Geometry: final body of the model. Coordinates: model frame, mm. Give positions to 0.01 mm unless a question says otherwise; leave off trailing zeros. Write each loop counter-clockwise with the first axis right and the second up, starting at its lowest first coordinate (ties: lowest second). Pieces come first, ordered by that corner, then holes. Notation, with made-up numbers: M 42,75.25 L 52,75.25 A22 cw 52,98.25 Z; hole C -20,86 d3. An arc over 180 degrees is marked long. One line per question, with ' | ' between items.
from build123d import *

# Parameters (mm, degrees)
F0_W     = 914.4
F0_H     = 762
F1_DEPTH = 609.6
F3_W     = 914.4
F3_H     = 762
F4_DEPTH = 609.6
F6_DEPTH = 2057.04989884
F8_DEPTH = 609.601


with BuildPart() as f1:
    # F0 (on Front) → F1 (new body)
    with BuildSketch(Plane.XZ):
        with Locations((-0.35110116, 123.4715153943)):
            Rectangle(F0_W, F0_H)
    extrude(amount=F1_DEPTH)


with BuildPart() as f1_1:
    # F2: moved
    add(f1.part.moved(Location((1143, 0, 0))))

    # F5 (on face) → F6 (cut, through all)
    with BuildSketch(Plane.YZ.offset(1599.84889884)):
        with BuildLine():
            Line((-609.6, 504.4715153943), (-609.6, -143.2284846057))
            ThreePointArc((-609.6, -143.2284846057), (-393.902496237, 149.2118568345), (-317.5, 504.4715153943))
            Line((-317.5, 504.4715153943), (-609.6, 504.4715153943))
        make_face()
    extrude(amount=-F6_DEPTH, mode=Mode.SUBTRACT)


with BuildPart() as f4:
    # F3 (on Front) → F4 (new body)
    with BuildSketch(Plane.XZ):
        Rectangle(F3_W, F3_H)
    extrude(amount=F4_DEPTH)

    # F7 (on face) → F8 (cut, through all)
    with BuildSketch(Plane.XZ.offset(609.6)):
        with BuildLine():
            Line((-457.2, 381), (-457.2, -266.7))
            ThreePointArc((-457.2, -266.7), (-287.4268495342, 37.5712410121), (-228.6, 381))
            Line((-228.6, 381), (-457.2, 381))
        make_face()
        with BuildLine():
            Line((457.2, 381), (228.6, 381))
            ThreePointArc((228.6, 381), (287.4268495342, 37.5712410121), (457.2, -266.7))
            Line((457.2, -266.7), (457.2, 381))
        make_face()
    extrude(amount=-F8_DEPTH, mode=Mode.SUBTRACT)


with BuildPart() as f1_2:
    # F9: moved
    add(f1_1.part.moved(Location((-1143, 0, -123.2408))))

    # F10: intersect F4
    add(f4.part, mode=Mode.INTERSECT)


solid = f1_2.part
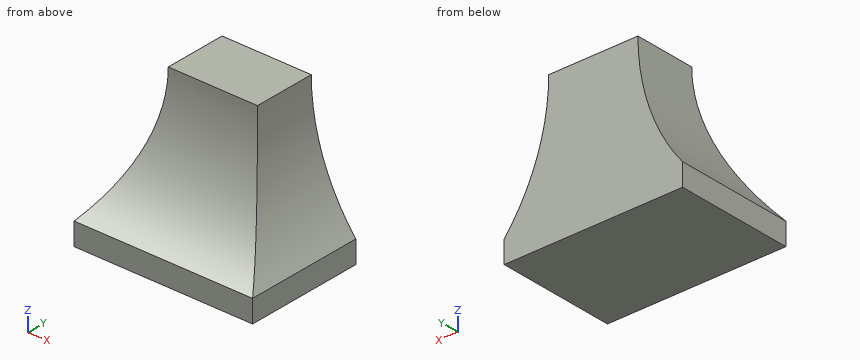
(1) Cut plane B-B, the plane y = -127. Return loops of the section in (x, z) (3 decimals), then the cut area to 3 significant figures.
Working result:
outline: M -457.2,-380.769 L 456.849,-380.769 L 456.849,-266.264 A1031.875 cw 228.6,381 L -228.6,381 A1031.875 cw -457.2,-266.7 Z | area: 494,000 mm^2
(2) Material intervals for L1, parallel to Z at x = 400.5, y = -110; L2, parallel to X at y = -108.5, z = 8; L3, parallel to Y at x = -215.5, z = -119.5, sorted ascending. Write a range as [from, to].
Working result:
L1: z = [-380.77, -189.27] | L2: x = [-298.37, 298.37] | L3: y = [-477.36, 0]
(3) First-contact query: P1, Ø3, axis at x = 76, y = -506.5, coming from the +Z side; P2, Ø1.5, axis at x = 96, z = -8, coming from the -Y side; P3, Ø12, axis at x = 266.5, z = 85.5, coming from the +Y side. Flat tips, straight axial feed; report the tip coordinate or a pass-through.
Working result:
P1: stops at z = -156.26 | P2: stops at y = -410.5 | P3: stops at y = 0
(4) Cut plane C-C, the plane z = 287. Return loops of the section in (x, y), then the cut area to 3 significant figures.
Working result:
outline: M -232.89,-322.65 L 232.89,-322.65 L 232.89,0 L -232.89,0 Z | area: 150,000 mm^2
(5) Cut plane D-D, the plane x = 295.5. Return loops of the section in (y, z), then the cut area to 3 significant figures.
Working result:
outline: M -609.6,-380.77 L 0,-380.77 L 0,15.5 L -398.71,15.5 A864.15 cw -609.6,-266.47 Z | area: 208,000 mm^2
(6) Cut plane A-A, the plane x = -16.5. Return loops of the section in (y, z).
Working result:
outline: M -609.6,-380.77 L 0,-380.77 L 0,381 L -317.5,381 A864.15 cw -609.6,-266.47 Z
